Can you work these out from the model? Positions are in its coordinate system, mm. Give positions to 0.01 mm unless a question says otherwise; leave off trailing zeros. Write each loop counter-clockwise with the first axis right and the second up, starting at its lowest first coordinate (ties: lowest second). Pieces come first, ordered by that corner, then holes. Notation, with made-up numbers: (66.5, 42.5) -> (96.5, 42.5) arc R14 ccw to (96.5, 49.5) -> close; hole circle Ø5 at (87.25, 78.5). An arc over 180 degrees is marked (long way). One line per item, written item: value.
from build123d import *

# Parameters (mm, degrees)
BOSS_EXTRUDE1_DEPTH = 469.9


with BuildPart() as part:
    # Sketch1 → Boss-Extrude1 (new body)
    with BuildSketch(Plane.XY):
        with BuildLine():
            Line((0, 2.54), (0, 38.1))
            Line((0, 38.1), (0.635, 38.1))
            ThreePointArc((0.635, 38.1), (2.431051224, 37.356051224), (3.175, 35.56))
            Line((3.175, 35.56), (3.175, 3.175))
            Line((3.175, 3.175), (35.56, 3.175))
            ThreePointArc((35.56, 3.175), (37.356051224, 2.431051224), (38.1, 0.635))
            Line((38.1, 0.635), (38.1, 0))
            Line((38.1, 0), (2.54, 0))
            ThreePointArc((2.54, 0), (0.743948776, 0.743948776), (0, 2.54))
        make_face()
    extrude(amount=BOSS_EXTRUDE1_DEPTH)


solid = part.part
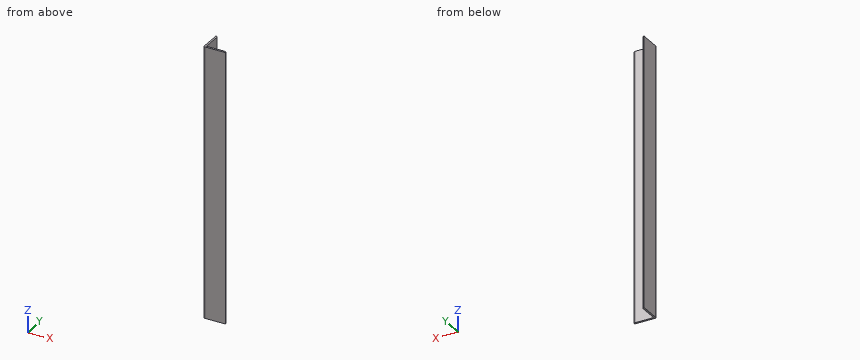
1) I need wall thicknesses on L1, parallel to X at y = 4, z = 175 (3 decimals); L2, parallel to X at y = 36, z = 336.5. Which ranges of each line are inside material? Lowest first, please.
Answer list:
L1: x = 0 to 3.175
L2: x = 0 to 3.14
2) Will these pins go through, and if not, where does the flat tip stop? pin 1 (3 mm diameter, centred on x = 5, y = 30, fed in from +Z); pin 2 (1.5 mm diameter, centred on x = 33, z = 110.5, fed in from +Y) (3 decimals); pin 3 (3 mm diameter, centred on y = 7.5, z = 333, fed in from +X) (3 decimals).
Answer list:
pin 1: passes through
pin 2: stops at y = 3.175
pin 3: stops at x = 3.175
3) If we section it at B-B (x = 20): Write out the boundary of the cut face in (y, z) (3 decimals), and give its area (3 significant figures).
Answer list:
outline: (0, 0) -> (3.175, 0) -> (3.175, 469.9) -> (0, 469.9) -> close
area: 1,490 mm^2
4) If we section it at A-A (z = 435.5): Write out the boundary of the cut face in (x, y) (3 decimals).
Answer list:
outline: (0, 2.54) arc R2.54 ccw to (2.54, 0) -> (38.1, 0) -> (38.1, 0.635) arc R2.54 ccw to (35.56, 3.175) -> (3.175, 3.175) -> (3.175, 35.56) arc R2.54 ccw to (0.635, 38.1) -> (0, 38.1) -> close
